Input: part model. Units: mm. Frame: model coordinates. Face numbers are marked on the shaded views. A direction names the side the tool comes from. Give positions to 0.01 mm unless a question says otherwise; leave off trailing zeros. Write each loop counter-clockwise with the first axis right and the second up, starting at its lowest first coordinate (ties: lowest second). Pieces come first, ordered by that corner, then holes. Notation, with made-up numbers: (88, 29.25) - (146, 29.25) arc R8 cw to (146, 40.25) - close; hole circle Ø9 at (54, -37). An arc over 180 degrees is marked (long way). Use a Markdown table: item, result. Add a question column.
1. Section query B-B, the plane z = 21.5. Return loops of the section in (x, y), plus the area to 3 significant figures.
2. Set-up query: the marked faces 1, 2, 3 and 4. Return all of +Z, -Z, +X, -X, +Y, -Y with unobstructed straight access to the full face (end or side cutting, diameter ignored); none if empty.
3. Pin query (flat end, axial travel): pin 1 (12 mm diameter, centred on x = 34.5, y = -64.5, fed in from +Z); pin 2 (3 mm diameter, centred on y = -70, z = 4, fed in from +X); pin 3 (6 mm diameter, centred on x = 20.5, y = -71.5, fed in from +Z). Return the tip coordinate at first contact, or that it passes through.
4. Material intervals for probe 1 along Z at (x, y) = (-11, 44); probe 2 along X at (y, z) = (32.5, 24.5); probe 3 along Y at (x, z) = (18, 48), sorted ascending.
5. Section query A-A, the plane y = 42.5. Return loops of the section in (x, z), plus the area to 3 significant figures.
```python
from build123d import *

# Parameters (mm, degrees)
F0_W      = 90
F0_H      = 55
F1_DEPTH  = 86
F2_DEPTH  = 12.5
F2_FACE_W = 90
F2_FACE_H = 55
F3_DEPTH  = 53.8
F4_DEPTH  = 65.3


with BuildPart() as f1:
    # F0 (on Front) → F1 (new body)
    with BuildSketch(Plane.XZ):
        with Locations((1.08182, -2.918677)):
            Rectangle(F0_W, F0_H)
    extrude(amount=F1_DEPTH)

    # F0 (on Front) → F2 (join, symmetric)
    with BuildSketch(Plane.XZ):
        with Locations((1.08182, -2.918677)):
            Rectangle(F0_W, F0_H)
    extrude(amount=F2_DEPTH, both=True)

    # F2_face (on face) → F3 (join)
    with BuildSketch(Plane(origin=(1.08182, 12.5, -2.918677), x_dir=(1, 0, 0), z_dir=(0, 1, 0))):
        Rectangle(F2_FACE_W, F2_FACE_H)
    extrude(amount=F3_DEPTH)

    # F0 (on Front) → F4 (join)
    with BuildSketch(Plane.XZ):
        with BuildLine():
            add(Edge.make_bspline(
                [(-43.91818, 24.581323), (-25.125932, 42.331356), (-13.193247, 60.789681), (66.08182, 57.259896)],
                knots=[0, 0, 0, 0, 114.751423, 114.751423, 114.751423, 114.751423], degree=3))
            Line((-43.91818, 24.581323), (46.08182, 24.581323))
            add(Edge.make_bspline(
                [(46.08182, 24.581323), (45.400707, 31.935), (61.706819, 30.563467), (66.08182, 32.259896)],
                knots=[0, 0, 0, 0, 21.423363, 21.423363, 21.423363, 21.423363], degree=3))
            Line((66.08182, 32.259896), (66.08182, 57.259896))
        make_face()
    extrude(amount=F4_DEPTH)


solid = f1.part
```
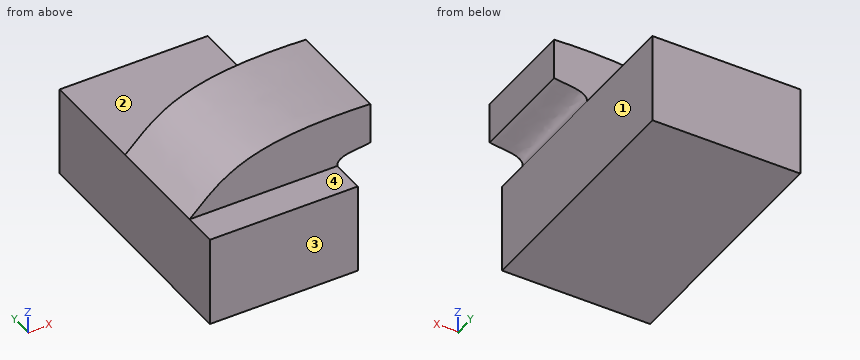
Result sheet:
| question | item | result |
|---|---|---|
| 1 | outline | (-43.92, -86) - (46.08, -86) - (46.08, 66.3) - (-43.92, 66.3) - close |
| 1 | area | 13,700 mm² |
| 2 | face 1 | -Z, +X, +Y, -Y |
| 2 | face 2 | +Z, +X, -X, +Y |
| 2 | face 3 | +Z, -Z, +X, -X, -Y |
| 2 | face 4 | +Z, +X, -X, -Y |
| 3 | pin 1 | stops at z = 57.62 |
| 3 | pin 2 | stops at x = 46.08 |
| 3 | pin 3 | stops at z = 24.58 |
| 4 | probe 1 | z = -30.42 to 24.58 |
| 4 | probe 2 | x = -43.92 to 46.08 |
| 4 | probe 3 | y = -65.3 to 0 |
| 5 | outline | (-43.92, -30.42) - (46.08, -30.42) - (46.08, 24.58) - (-43.92, 24.58) - close |
| 5 | area | 4,950 mm² |
